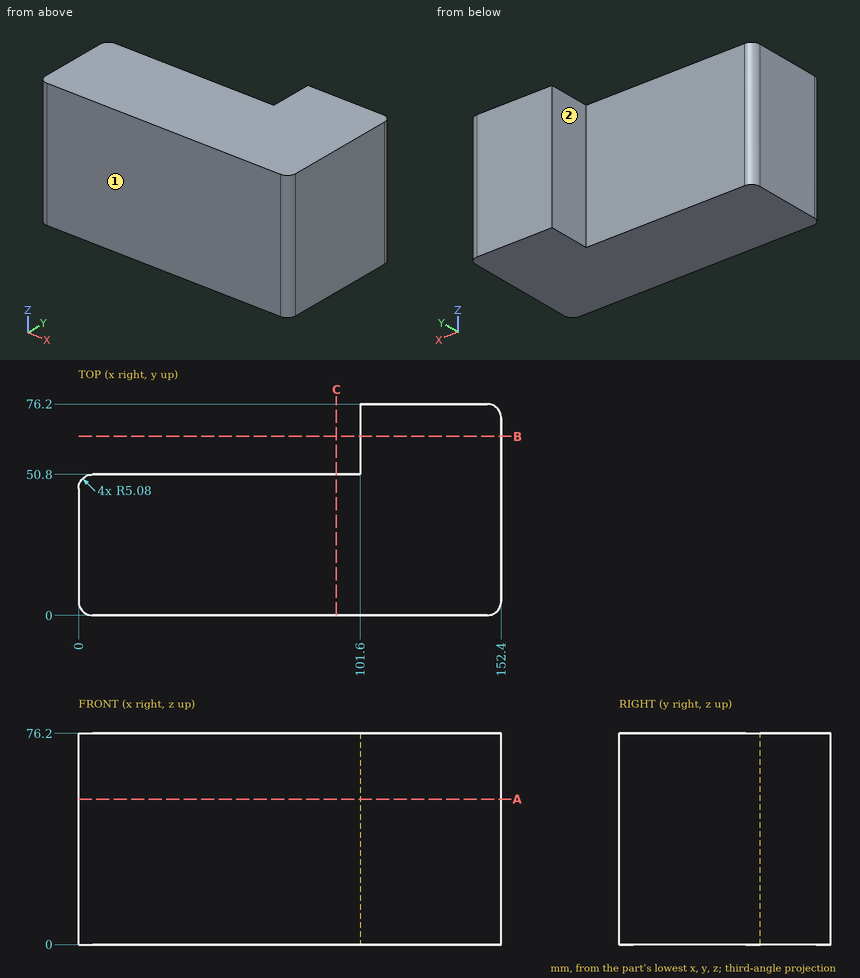
For this review, use the dimensioned drawing (mm, ordinates from the lowest corner) and the shaded views. A direction names the side the tool comes from. Round coordinates to 2 decimals unless told otherwise and drop trailing zeros. Write each loop counter-clockwise with the first axis right and the second up, starting at its lowest first coordinate (ties: lowest second). Pieces come first, ordered by that corner, then holes. Notation, with made-up numbers: (1.5, -19.5) - (16.5, -19.5) arc R31 cw to (16.5, 19.5) - close; hole circle Ø8 at (-22.75, 89). An arc over 180 degrees is marked (long way). Answer as a JSON object with one key per item and string values.
1. We need section C-C on x = 93. Give the boundary of the cut face in (y, z), then the cut area to 3 significant figures.
Response values:
{"outline": "(0, 0) - (50.8, 0) - (50.8, 76.2) - (0, 76.2) - close", "area": "3,870 mm2"}
2. We need section A-A on z = 52.5. Give the boundary of the cut face in (x, y).
Response values:
{"outline": "(0, 5.08) arc R5.08 ccw to (5.08, 0) - (147.32, 0) arc R5.08 ccw to (152.4, 5.08) - (152.4, 71.12) arc R5.08 ccw to (147.32, 76.2) - (101.6, 76.2) - (101.6, 50.8) - (5.08, 50.8) arc R5.08 ccw to (0, 45.72) - close"}
3. To check wall thickness, follow line 1 along Y through (x, z) = (67, 10); line 2 along X through (y, z) = (52, 32); line 3 along X through (y, z) = (47, 17). State the ranges of each line that lie inside material, in increasing order.
Response values:
{"line 1": "y = 0 to 50.8", "line 2": "x = 101.6 to 152.4", "line 3": "x = 0.16 to 152.4"}
4. We need section B-B on y = 64.5. Give the boundary of the cut face in (x, z), then the cut area to 3 significant figures.
Response values:
{"outline": "(101.6, 0) - (152.4, 0) - (152.4, 76.2) - (101.6, 76.2) - close", "area": "3,870 mm2"}
5. For pin 1 Ø8 at (x, z) = (33, 62.5) entering from +Y, flat-tipped, find the tip position at first contact; note if it passes through.
Response values:
{"pin 1": "stops at y = 50.8"}
6. Tool access review of the marked faces 1 and 2: name each direction out of +Z, -Z, +X, -X, +Y, -Y from which nothing blocks a thin tool from reaching the whole face with its end or side.
Response values:
{"face 1": "+Z, -Z, +X, -X, -Y", "face 2": "+Z, -Z, -X, +Y"}
